Design review of the part built by this model. Coordinates are the model's own, in mm. A direction names the side the tool comes from. Give positions to 0.01 mm unless a question says otherwise; leave off trailing zeros. Loops run counter-clockwise (first coordinate to the right, second up) from the corner with the lowest first, then second, coordinate; pieces in that order, holes last. Notation, with made-up numbers: (-17, 11.25) -> (-4, 11.25) arc R22 ccw to (-4, 32.25) -> close; hole circle Ø7 at (-6, 16). An arc over 180 degrees is marked (long way). Use a Markdown table: item, result. Add a question column.
1. Draft analysis for pull direction Y (two halves, no side actions). For faces 1 (the flat face through (0, 4.762, 3)), 2 (the flat face through (-18.64, 1.95, 1.04)), 3 (the cylindrical face through (-21.394, -0.105, 3.131)), 4 (the flat face through (-14.68, 2.01, 1.04)), state which applies: pulls with the +Y half, pulls with the -Y half, needs draft (parallel to the pull), parting line crosses it, or undercut.
2. Add section A-A (z = 5). Count the separate pieces of the cut face and the enclosed holes in it, and give its area (3 significant figures).
3. Add section B-B (y = -1.25). State the section outline as (x, z) points.
4. To check wall thickness, follow line 1 (X direction, y = 0.5, z = 3.5); line 2 (X direction, y = 2.5, z = 1); line 3 (X direction, y = 1.5, z = 2). State the ranges of each line that lie inside material, in increasing order.
5. For faces 5 (the flat face through (0, -4.762, 3)), 6 (the flat face through (-14.627, -1.955, 1.035)), list the 3-axis set-ups (+Z, -Z, +X, -X, +Y, -Y) from which the entire face can be reached by the end or side of a thin tool; tool diameter is ignored.
```python
from build123d import *

# Parameters (mm, degrees)
SKETCH1_R           = 1.65
BOSS_EXTRUDE1_DEPTH = 6.35
CUT_EXTRUDE1_DEPTH  = 2.1
FILLET1_R           = 0.254


with BuildPart() as part:
    # Sketch1 → Boss-Extrude1 (new body)
    with BuildSketch(Plane.XY):
        with BuildLine():
            Line((-16.632351927, 4.7625), (16.632351927, 4.7625))
            ThreePointArc((16.632351927, 4.7625), (21.394851927, 0), (16.632351927, -4.7625))
            Line((16.632351927, -4.7625), (-16.632351927, -4.7625))
            ThreePointArc((-16.632351927, -4.7625), (-21.394851927, 0), (-16.632351927, 4.7625))
        make_face()
        with Locations((16.632351927, 0)):
            Circle(SKETCH1_R, mode=Mode.SUBTRACT)
        with Locations((-16.632351927, 0)):
            Circle(SKETCH1_R, mode=Mode.SUBTRACT)
    extrude(amount=BOSS_EXTRUDE1_DEPTH)

    # Sketch2 → Cut-Extrude1 (cut)
    with BuildSketch(Plane(origin=(0, 0, 0), x_dir=(-1, 0, 0), z_dir=(0, 0, -1))):
        Polygon((12.672553952, 0), (16.632351927, -3.959797975), (20.592149902, 0), (16.632351927, 3.959797975), align=None)
    extrude(amount=-CUT_EXTRUDE1_DEPTH, mode=Mode.SUBTRACT)

    # Fillet1
    fillet1_edges = [part.edges().sort_by_distance(p)[0] for p in [
        (-20.592149902, 0, 1.05),
        (-16.632351927, -3.959797975, 1.05),
        (-12.672553952, 0, 1.05),
        (-16.632351927, 3.959797975, 1.05),
    ]]
    fillet(fillet1_edges, radius=FILLET1_R)


solid = part.part
```
Taken from the geometry:
| question | item | result |
|---|---|---|
| 1 | face 1 | pulls with the +Y half |
| 1 | face 2 | undercut |
| 1 | face 3 | parting line crosses it |
| 1 | face 4 | undercut |
| 2 | separate pieces | 1 |
| 2 | enclosed holes | 2 |
| 2 | area | 371 mm^2 |
| 3 | outline | (-21.23, 0) -> (-19.34, 0) -> (-19.34, 2.1) -> (-17.71, 2.1) -> (-17.71, 6.35) -> (-21.23, 6.35) -> close; (-15.56, 2.1) -> (-13.92, 2.1) -> (-13.92, 0) -> (15.56, 0) -> (15.56, 6.35) -> (-15.56, 6.35) -> close; (17.71, 0) -> (21.23, 0) -> (21.23, 6.35) -> (17.71, 6.35) -> close |
| 4 | line 1 | x = -21.37 to -18.2, -15.06 to 15.06, 18.2 to 21.37 |
| 4 | line 2 | x = -20.69 to -18.09, -15.17 to 20.69 |
| 4 | line 3 | x = -21.15 to -19.09, -14.17 to 15.94, 17.32 to 21.15 |
| 5 | face 5 | +Z, -Z, +X, -X, -Y |
| 5 | face 6 | -Z |
